Can you work these out from the model? Positions are in its coordinate system, mm. Give positions to 0.01 mm unless a question says otherwise; leave off trailing zeros. Loops run counter-clockwise (first coordinate to the right, second up) from the corner with the lowest first, then second, coordinate; pieces in that order, holes last. Notation, with made-up numbers: (-29.75, 40.5) - (-0.75, 40.5) arc R21 ccw to (-0.75, 76.5) - close; hole circle Ø8 at (67, 12.25). An arc over 180 degrees is marked (long way). Answer as a JSON object with one key per item and string values.
```python
from build123d import *

# Parameters (mm, degrees)
BOSS_EXTRUDE2_DEPTH = 6.35
CUT_EXTRUDE1_DEPTH  = 7.3500001
BOSS_EXTRUDE3_DEPTH = 6.35
SKETCH10_R          = 3.96875
CUT_EXTRUDE2_DEPTH  = 7.35
SKETCH11_R          = 4.5
CUT_EXTRUDE4_DEPTH  = 7.35
BOSS_EXTRUDE4_DEPTH = 6.35
SKETCH13_R          = 1.75
CUT_EXTRUDE5_DEPTH  = 7.35
LPATTERN1_COUNT     = 2
LPATTERN1_PITCH     = 64
SKETCH15_R          = 1.75
CUT_EXTRUDE7_DEPTH  = 7.35
SKETCH16_R          = 1.75
CUT_EXTRUDE8_DEPTH  = 7.35
SKETCH17_R          = 1.75
CUT_EXTRUDE9_DEPTH  = 7.35
SKETCH18_R          = 1.75
SKETCH18_R_2        = 6.35
CUT_EXTRUDE10_DEPTH = 7.35
CUT_EXTRUDE11_DEPTH = 7.35
CUT_EXTRUDE12_DEPTH = 7.35
FILLET1_R           = 3.175
FILLET2_R           = 3.175


with BuildPart() as part:
    # Sketch6 → Boss-Extrude2 (new body)
    with BuildSketch(Plane.XY):
        with BuildLine():
            Line((-68.006850091, -76.67090114), (-109.486767671, -48.656527855))
            Line((-109.486767671, -48.656527855), (-118.371760678, -61.812230963))
            Line((-118.371760678, -61.812230963), (18.447551645, -154.216158235))
            Line((18.447551645, -154.216158235), (135.729459338, 19.43912279))
            Line((135.729459338, 19.43912279), (-1.089852986, 111.843050063))
            Line((-1.089852986, 111.843050063), (-73.946795643, 3.966284577))
            Line((-73.946795643, 3.966284577), (-56.624438948, -7.732749433))
            ThreePointArc((-56.624438948, -7.732749433), (-43.058385537, 37.577891571), (0, 57.15))
            ThreePointArc((0, 57.15), (56.404848571, 31.095576642), (70.829334649, -29.338471048))
            add(Edge.make_bspline(
                [(70.829334649, -29.338471048), (70.811686062, -29.418295928), (70.776015112, -29.578104383), (70.713320217, -29.85478305), (70.619021771, -30.262929245), (70.501052001, -30.762086912), (70.364034474, -31.322191481), (70.199318515, -31.970958926), (70.000453855, -32.723919765), (69.795103485, -33.469783355), (69.582015398, -34.214296028), (69.361377803, -34.956693289), (69.133257682, -35.696762218), (68.838782679, -36.61892651), (68.470566207, -37.720710028), (68.019498024, -38.998776477), (67.474836154, -40.448808619), (66.901337925, -41.887676852), (66.299328392, -43.31485223), (65.669141732, -44.729810424), (65.011119088, -46.132040323), (64.325609411, -47.52103904), (63.612968547, -48.896314904), (62.87355937, -50.257385735), (62.107751613, -51.603779381), (61.315921169, -52.935034173), (60.49845004, -54.250698756), (59.655726138, -55.550331897), (58.571247582, -57.154294757), (57.220953058, -59.045283389), (55.576035723, -61.200397094), (53.604026134, -63.590264702), (51.54329346, -65.904053004), (49.39728314, -68.138962994), (47.169496434, -70.29235602), (44.863486103, -72.361752995), (42.482847363, -74.344831806), (40.031215607, -76.239428526), (36.882516177, -78.494556171), (32.976808929, -81.016011003), (28.250788286, -83.68089187), (21.41551215, -86.919136497), (14.30829026, -89.526654921), (6.996956895, -91.488176442), (-0.451922312, -92.797413176), (-6.61686174, -93.456358442), (-12.81195397, -93.702029749), (-19.009644204, -93.537285056), (-25.183124422, -92.966685286), (-31.306438312, -91.996382122), (-36.598524037, -90.804323442), (-41.072542301, -89.543185606), (-44.752319298, -88.33589156), (-47.664184976, -87.27761875), (-50.541347258, -86.128353728), (-53.381128552, -84.889612663), (-56.180924218, -83.562977818), (-58.593536599, -82.326710176), (-60.633378351, -81.214215821), (-62.313751085, -80.252471782), (-63.646071553, -79.462491566), (-64.966093336, -78.652178853), (-66.222359154, -77.854259082), (-67.143044791, -77.250601571), (-67.736251212, -76.85365602), (-68.006850091, -76.67090114)],
                knots=[0.071020771, 0.071020771, 0.071020771, 0.071020771, 0.071020771, 0.072848477, 0.074676184, 0.07650389, 0.078331597, 0.08198701, 0.085642423, 0.089297836, 0.092953249, 0.096608662, 0.100264075, 0.103919488, 0.107574901, 0.114885727, 0.122196554, 0.12950738, 0.136818214, 0.144129048, 0.151439882, 0.158750716, 0.166061558, 0.173372401, 0.180683243, 0.187994085, 0.195304924, 0.202615763, 0.209926602, 0.217237441, 0.231859103, 0.246480766, 0.261102426, 0.275724085, 0.290345754, 0.304967424, 0.319589099, 0.334210774, 0.348832457, 0.36345414, 0.392697464, 0.421940789, 0.451184112, 0.506140643, 0.535383973, 0.564627303, 0.593870641, 0.623113979, 0.652357319, 0.68160066, 0.710843985, 0.740087309, 0.754708984, 0.769330659, 0.783952333, 0.798574008, 0.813195669, 0.82781733, 0.842438991, 0.849749821, 0.857060652, 0.86437149, 0.871682327, 0.878993165, 0.885158103, 0.885158103, 0.885158103, 0.885158103, 0.885158103], degree=4))
        make_face()
    extrude(amount=BOSS_EXTRUDE2_DEPTH)

    # Sketch8 → Cut-Extrude1 (cut, through all)
    with BuildSketch(Plane.XY.offset(6.35)):
        Polygon((-71.011229489, -93.798205788), (-53.378672597, -90.381637707), (-42.854110111, -97.489632113), (-39.43754203, -115.122189004), align=None)
    extrude(amount=-CUT_EXTRUDE1_DEPTH, mode=Mode.SUBTRACT)

    # Sketch9 → Boss-Extrude3 (add, through all)
    with BuildSketch(Plane.XY.offset(6.35)):
        Polygon((-1.089852986, 111.843050063), (-109.486767671, -48.656527855), (27.332544652, -141.060455127), (135.729459338, 19.43912279), align=None)
    extrude(amount=-BOSS_EXTRUDE3_DEPTH)

    # Sketch10 → Cut-Extrude2 (cut, through all)
    with BuildSketch(Plane.XY.offset(6.35)):
        with Locations((4.996496209, -84.796642912)):
            Circle(SKETCH10_R)
        with Locations((40.816310536, -31.759477627)):
            Circle(SKETCH10_R)
        with Locations((76.636124864, 21.277687659)):
            Circle(SKETCH10_R)
        with Locations((-45.295165913, -45.214466102)):
            Circle(SKETCH10_R)
    extrude(amount=-CUT_EXTRUDE2_DEPTH, mode=Mode.SUBTRACT)

    # Sketch11 → Cut-Extrude4 (cut, through all)
    with BuildSketch(Plane.XY.offset(6.35)):
        Circle(SKETCH11_R)
    extrude(amount=-CUT_EXTRUDE4_DEPTH, mode=Mode.SUBTRACT)

    # Sketch12 → Boss-Extrude4 (add, through all)
    with BuildSketch(Plane.XY.offset(6.35)):
        Polygon((135.729459338, 19.43912279), (67.319803176, 65.641086427), (88.643786393, 97.214773886), (157.053442554, 51.01281025), align=None)
    extrude(amount=-BOSS_EXTRUDE4_DEPTH)

    # Sketch13 → Cut-Extrude5 (cut, through all)
    with BuildSketch(Plane.XY.offset(6.35)):
        with Locations((94.899221836, -29.671127724)):
            Circle(SKETCH13_R)
    cut_extrude5 = extrude(amount=-CUT_EXTRUDE5_DEPTH, mode=Mode.SUBTRACT)

    # LPattern1: Cut-Extrude5 ×2
    with Locations(*[Vector(-0.559684599, -0.828705708, 0) * (i * LPATTERN1_PITCH) for i in range(1, LPATTERN1_COUNT)]):
        add(cut_extrude5, mode=Mode.SUBTRACT)

    # Sketch15 → Cut-Extrude7 (cut, through all)
    with BuildSketch(Plane.XY.offset(6.35)):
        with Locations((-105.147343009, -59.249804902)):
            Circle(SKETCH15_R)
        with Locations((15.885125585, -140.991740566)):
            Circle(SKETCH15_R)
        with Locations((1.472573075, 98.618632394)):
            Circle(SKETCH15_R)
    extrude(amount=-CUT_EXTRUDE7_DEPTH, mode=Mode.SUBTRACT)

    # Sketch16 → Cut-Extrude8 (cut, through all)
    with BuildSketch(Plane.XY.offset(6.35)):
        with Locations((92.060354474, 79.582216994)):
            Circle(SKETCH16_R)
        with Locations((139.420885662, 47.596242169)):
            Circle(SKETCH16_R)
    extrude(amount=-CUT_EXTRUDE8_DEPTH, mode=Mode.SUBTRACT)

    # Sketch17 → Cut-Extrude9 (cut, through all)
    with BuildSketch(Plane.XY.offset(6.35)):
        with Locations((-26.311406216, 17.769986014)):
            Circle(SKETCH17_R)
        with Locations((17.769986014, 26.311406216)):
            Circle(SKETCH17_R)
    extrude(amount=-CUT_EXTRUDE9_DEPTH, mode=Mode.SUBTRACT)

    # Sketch18 → Cut-Extrude10 (cut, through all)
    with BuildSketch(Plane.XY.offset(6.35)):
        with Locations((75.468896753, 66.798604333)):
            Circle(SKETCH18_R)
        with Locations((74.378499235, 51.337005669)):
            Circle(SKETCH18_R)
        with Locations((87.223437703, 42.661894386)):
            Circle(SKETCH18_R)
        with Locations((101.158773688, 49.448381768)):
            Circle(SKETCH18_R)
        with Locations((102.249171205, 64.909980432)):
            Circle(SKETCH18_R)
        with Locations((89.404232738, 73.585091715)):
            Circle(SKETCH18_R)
        with Locations((99.589076537, 21.914747078)):
            Circle(SKETCH18_R)
        with Locations((104.266720973, 36.692082512)):
            Circle(SKETCH18_R)
        with Locations((119.403091077, 40.029791318)):
            Circle(SKETCH18_R)
        with Locations((129.861816745, 28.59016469)):
            Circle(SKETCH18_R)
        with Locations((125.18417231, 13.812829255)):
            Circle(SKETCH18_R)
        with Locations((110.047802206, 10.47512045)):
            Circle(SKETCH18_R)
        with Locations((105.180381325, -7.122099496)):
            Circle(SKETCH18_R)
        with Locations((96.077150237, 5.423066257)):
            Circle(SKETCH18_R)
        with Locations((80.661102457, 3.812019754)):
            Circle(SKETCH18_R)
        with Locations((74.348285765, -10.344192501)):
            Circle(SKETCH18_R)
        with Locations((83.451516853, -22.889358254)):
            Circle(SKETCH18_R)
        with Locations((98.867564633, -21.278311751)):
            Circle(SKETCH18_R)
        with Locations((84.396043028, 52.322553097)):
            Circle(SKETCH18_R_2)
        with Locations((108.051811284, 27.364940468)):
            Circle(SKETCH18_R_2)
        with Locations((95.429892272, -4.622009378)):
            Circle(SKETCH18_R_2)
    extrude(amount=-CUT_EXTRUDE10_DEPTH, mode=Mode.SUBTRACT)

    # Sketch19 → Cut-Extrude11 (cut, through all)
    with BuildSketch(Plane.XY.offset(6.35)):
        Polygon((67.319803176, 65.641086427), (-1.089852986, 111.843050063), (-118.81528907, -62.468948176), (-50.405632909, -108.670911813), align=None)
    extrude(amount=-CUT_EXTRUDE11_DEPTH, mode=Mode.SUBTRACT)

    # Sketch20 → Cut-Extrude12 (cut, through all)
    with BuildSketch(Plane.XY.offset(6.35)):
        Polygon((85.800588631, 93.004948891), (87.167215863, 85.951926135), (71.529628171, 62.797888664), (67.319803176, 65.641086427), align=None)
    extrude(amount=-CUT_EXTRUDE12_DEPTH, mode=Mode.SUBTRACT)

    # Fillet1
    fillet1_edges = [part.edges().sort_by_distance(p)[0] for p in [
        (18.447551645, -154.216158235, 3.175),
        (87.167215863, 85.951926135, 3.175),
        (85.800588631, 93.004948891, 3.175),
        (71.529628171, 62.797888664, 3.175),
        (-39.43754203, -115.122189004, 3.175),
        (-42.854110111, -97.489632113, 3.175),
        (157.053442554, 51.01281025, 3.175),
        (88.643786393, 97.214773886, 3.175),
    ]]
    fillet(fillet1_edges, radius=FILLET1_R)

    # Fillet2
    fillet2_edges = [part.edges().sort_by_distance(p)[0] for p in [
        (67.319803176, 65.641086427, 3.175),
    ]]
    fillet(fillet2_edges, radius=FILLET2_R)


solid = part.part
```
1) Imagine slicing it at B-B on z = 3.75. Give the number of separate pieces and of enclosed holes in the cut face, and give its area (3 significant figures).
Check sheet entries:
{"separate pieces": "1", "enclosed holes": "28", "area": "19,500 mm2"}
2) If we mould it in two halves opening along X, with no side actions, what happens to faces 1 (the flat face through (58, -27, 6.35)), 2 (the flat face through (122.41, 74.41, 3.22)), 3 (the cylindrical face through (39.956, -35.634, 3.219)), 4 (the cylindrical face through (72.67, 21.45, 3.22))? For each: released by +X, released by -X, zero draft, split by the parting line, or undercut.
Check sheet entries:
{"face 1": "zero draft", "face 2": "released by +X", "face 3": "undercut", "face 4": "undercut"}
3) Imagine slicing it at A-A on x = -4.5. Write out the boundary of the cut face in (y, z), and give its area (3 significant figures).
Check sheet entries:
{"outline": "(-138.72, 0) - (-40.7, 0) - (-40.7, 6.35) - (-138.72, 6.35) - close", "area": "622 mm2"}
4) I'm going to push flat-ended pins straight in: P1, Ø7.5, axis at x = 84.4, y = 52.32, coming from the -Z side; P2, Ø1.5, axis at y = -25, z = 4.5, coming from the +X side; P3, Ø1, axis at y = -9.5, z = 4, coming from the -X side. Where does each tip first touch, or does it pass through?
Check sheet entries:
{"P1": "through", "P2": "x = 106.22", "P3": "x = 16.23"}
5) Imagine slicing it at C-C on y = -63. Write out the boundary of the cut face in (x, z).
Check sheet entries:
{"outline": "(-19.56, 0) - (80.05, 0) - (80.05, 6.35) - (-19.56, 6.35) - close"}
6) I need wall thicknesses on L1, parallel to X at y = -82, z = 4.75; L2, parallel to X at y = -10, z = 3; L3, parallel to Y at x = 94, z = 2. Which ranges of each line are inside material? Lowest first, please.
Check sheet entries:
{"L1": "-32.39 to 2.18, 7.81 to 57.48, 60.68 to 67.22", "L2": "16.23 to 72.63, 76.06 to 92.05, 98.81 to 115.85", "L3": "-42.35 to -31.17, -28.17 to -10.81, 1.56 to 93.6"}
